```python
from build123d import *

# Parameters (mm, degrees)
F1_DEPTH = 20
F2_R     = 7.5
F3_DEPTH = 20
F4_R     = 7


with BuildPart() as f1:
    # F0 (on Top) → F1 (new body)
    with BuildSketch(Plane.XY):
        with BuildLine():
            ThreePointArc((9.682458, 17.5), (0, 20), (-9.682458, 17.5))
            Line((-9.682458, 17.5), (9.682458, 17.5))
        make_face()
    extrude(amount=F1_DEPTH)

    # F2 (on face) → F3 (join)
    with BuildSketch(Plane.XZ.offset(-17.5)):
        with Locations((0, 10)):
            Circle(F2_R)
    extrude(amount=-F3_DEPTH)

    # F4
    f4_edges = [f1.edges().sort_by_distance(p)[0] for p in [
        (-7.5, 37.5, 10),
    ]]
    fillet(f4_edges, radius=F4_R)


solid = f1.part
```
Design review of the part built by this model. Coordinates are the model's own, in mm. A direction names the side the tool comes from. Round coordinates to 2 decimals unless told otherwise and drop trailing zeros. Order: outer loops, then holes, each group sorted by start corner. A loop starts at its lowest first (then second) coordinate and runs counter-clockwise, first axis right, second up. Notation, with made-up numbers: (56.25, 66.25) - (92.25, 66.25) arc R12 cw to (92.25, 89.25) - close; hole circle Ø3 at (-22.75, -37). An arc over 180 degrees is marked (long way). One line per question, with ' | ' between items.
Item 1: For P1, Ø6, axis at x = 7, y = 34.5, coming from the -Z side; P2, Ø3, axis at x = 3, y = 23.5, coming from the -Z side; P3, Ø3, axis at y = 34, z = 16, coming from the -X side, all flat-tipped, find the tip position at first contact; note any pin that passes through.
Checks:
P1: z = 4.51 | P2: z = 2.65 | P3: x = -5.1
Item 2: Machinability: for faces 1 (the face through (-1.63, 24.44, 2.68)), 2 (the face through (0, 18, 20)), which of the approach directions +Z, -Z, +X, -X, +Y, -Y give a long, thin tool a straight path to every point of the face, cutting with its end or side? Answer none if there is none.
Checks:
face 1: +Y | face 2: +Z, +X, -X, +Y, -Y
Item 3: Wall thickness on line 1 (Z direction, x = -6.5, y = 25); line 2 (Y direction, x = 1.75, z = 6.5); line 3 (X direction, y = 22.75, z = 11.75): over which ranges is each line inside the solid? List them lowest first. Write a range as [from, to].
Checks:
line 1: [6.26, 13.74] | line 2: [17.5, 36.61] | line 3: [-7.29, 7.29]
Item 4: Take a section at A-A, the plane y = 28.25. Write out the cut boundary in (x, z), then the cut area to 3 significant figures.
Checks:
outline: circle Ø15 at (0, 10) | area: 177 mm²
